```python
from build123d import *

# Parameters (mm, degrees)
F0_R     = 14.2875
F1_DEPTH = 15.875


# Not quite as in the source:
# - a length typed as a fraction of an inch, garbled in the dataset ("3 / 203.2 mm" for 3/8 in), is restored
# - a feature names something its author has since deleted; it is built from what else it names


with BuildPart() as f1:
    # F0 (on Front) → F1 (new body)
    with BuildSketch(Plane.XZ):
        with BuildLine():
            Line((25.4, 22), (-25.4, 22))
            ThreePointArc((-25.4, 22), (-40.9563491861, 15.5563491861), (-47.4, 0))
            ThreePointArc((-47.4, 0), (-40.9563491861, -15.5563491861), (-25.4, -22))
            Line((-25.4, -22), (25.4, -22))
            ThreePointArc((25.4, -22), (40.9563491861, -15.5563491861), (47.4, 0))
            ThreePointArc((47.4, 0), (40.9563491861, 15.5563491861), (25.4, 22))
        make_face()
        with Locations((-25.4, 0)):
            Circle(F0_R, mode=Mode.SUBTRACT)
        with Locations((25.4, 0)):
            Circle(F0_R, mode=Mode.SUBTRACT)
    extrude(amount=F1_DEPTH)


solid = f1.part
```
Build history of the part. All positions in model axes, mm. Round coordinates to 2 decimals unless told otherwise and drop trailing zeros. Write each loop counter-clockwise with the first axis right and the second up, starting at its lowest first coordinate (ties: lowest second). Pieces come first, ordered by that corner, then holes. Notation, with made-up numbers: (39.25, -1) -> (45.25, -1) arc R32 ccw to (45.25, 37) -> close; hole circle Ø4 at (-6.75, 58.25). An arc over 180 degrees is marked (long way). Put each result on its own line as item: value.
Item 1: Slice it at A-A, the plane y = -7.75. Give the cut face in (x, z) (1 decimal).
Here are the results:
outline: (-25.4, -22) -> (25.4, -22) arc R22 ccw to (25.4, 22) -> (-25.4, 22) arc R22 ccw to start; hole circle Ø28.6 at (-25.4, 0); hole circle Ø28.6 at (25.4, 0)
Item 2: Flat gauge pins, fed straight in: P1, Ø12, axis at x = 35, z = 6.5, coming from the -Y side (3 decimals); P2, Ø4, axis at x = 31, y = -9.5, coming from the +Z side; P3, Ø3, axis at y = -8.5, z = -9, coming from the -X side; P4, Ø5, axis at y = -11.5, z = 3, coming from the -X side. Where does each tip first touch, or does it go through?
Here are the results:
P1: stops at y = -15.875
P2: stops at z = 21.7
P3: stops at x = -46.08
P4: stops at x = -47.39
Item 3: Wall check: probe 1 along X at (y, z) = (-4.25, 7); probe 2 along Z at (x, y) = (25.4, -5.5); probe 3 along X at (y, z) = (-2, 6.5). Give the ranges that are in metal, low to high. Write a range as from..to.
Here are the results:
probe 1: x = -46.26..-37.86, -12.94..12.94, 37.86..46.26
probe 2: z = -22..-14.29, 14.29..22
probe 3: x = -46.42..-38.12, -12.68..12.68, 38.12..46.42
Item 4: Slice it at D-D, the plane x = -30.5. Give the cut face in (y, z) (3 decimals).
Here are the results:
outline: (-15.875, -21.401) -> (0, -21.401) -> (0, -13.346) -> (-15.875, -13.346) -> close; (-15.875, 13.346) -> (0, 13.346) -> (0, 21.401) -> (-15.875, 21.401) -> close
Item 5: Slice it at B-B, the plane x = 18. Give the cut face in (y, z) (3 decimals), plus the area to 3 significant figures.
Here are the results:
outline: (-15.875, -22) -> (0, -22) -> (0, -12.222) -> (-15.875, -12.222) -> close; (-15.875, 12.222) -> (0, 12.222) -> (0, 22) -> (-15.875, 22) -> close
area: 310 mm^2
Item 6: Slice it at C-C, the plane z = -7. Give the cut face in (x, y) (3 decimals).
Here are the results:
outline: (-46.257, -15.875) -> (-37.855, -15.875) -> (-37.855, 0) -> (-46.257, 0) -> close; (-12.945, -15.875) -> (12.945, -15.875) -> (12.945, 0) -> (-12.945, 0) -> close; (37.855, -15.875) -> (46.257, -15.875) -> (46.257, 0) -> (37.855, 0) -> close
